Verification items for the finished model (mm, model axes). Face numbers are marked on the shaded views. A direction names the side the tool comes from. Give positions to 0.01 mm unless a question says otherwise; leave off trailing zeros. Write each loop counter-clockwise with the first axis right and the second up, starting at its lowest first coordinate (ties: lowest second). Pieces come first, ordered by that corner, then holes. Notation, with made-up numbers: (43.25, 46.5) -> (71.25, 46.5) arc R10 cw to (71.25, 60.5) -> close; hole circle Ø9 at (19, 47). An arc over 180 degrees is marked (long way). Answer as CSV lines item,"result".
```python
from build123d import *

# Parameters (mm, degrees)
BOSS_EXTRUDE1_DEPTH = 10
SKETCH4_R           = 4
CUT_EXTRUDE1_DEPTH  = 11


with BuildPart() as part:
    # Sketch3 → Boss-Extrude1 (new body)
    with BuildSketch(Plane.XY):
        with BuildLine():
            Line((-13.081475452, 10.960155108), (-10.960155108, 8.838834765))
            Line((-10.960155108, 8.838834765), (-10.960155108, -8.838834765))
            Line((-10.960155108, -8.838834765), (-13.081475452, -10.960155108))
            ThreePointArc((-13.081475452, -10.960155108), (-13.081475452, -13.081475452), (-10.960155108, -13.081475452))
            Line((-10.960155108, -13.081475452), (-8.838834765, -10.960155108))
            Line((-8.838834765, -10.960155108), (8.838834765, -10.960155108))
            Line((8.838834765, -10.960155108), (10.960155108, -13.081475452))
            ThreePointArc((10.960155108, -13.081475452), (13.081475452, -13.081475452), (13.081475452, -10.960155108))
            Line((13.081475452, -10.960155108), (10.960155108, -8.838834765))
            Line((10.960155108, -8.838834765), (10.960155108, 8.838834765))
            Line((10.960155108, 8.838834765), (13.081475452, 10.960155108))
            ThreePointArc((13.081475452, 10.960155108), (13.081475452, 13.081475452), (10.960155108, 13.081475452))
            Line((10.960155108, 13.081475452), (8.838834765, 10.960155108))
            Line((8.838834765, 10.960155108), (-8.838834765, 10.960155108))
            Line((-8.838834765, 10.960155108), (-10.960155108, 13.081475452))
            ThreePointArc((-10.960155108, 13.081475452), (-13.081475452, 13.081475452), (-13.081475452, 10.960155108))
        make_face()
    extrude(amount=-BOSS_EXTRUDE1_DEPTH)

    # Sketch4 → Cut-Extrude1 (cut, through all)
    with BuildSketch(Plane.XY):
        Circle(SKETCH4_R)
    extrude(amount=-CUT_EXTRUDE1_DEPTH, mode=Mode.SUBTRACT)


solid = part.part
```
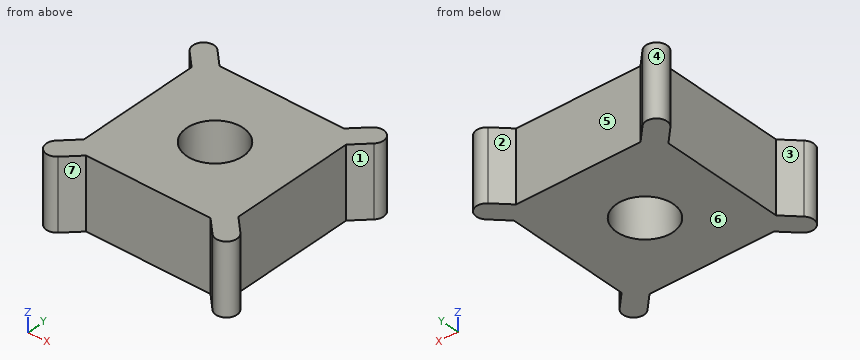
1) Section check A-A (y = 0). Record the boundary of the cut face in (x, z), and give its area (3 significant figures).
Reported:
outline,"(-10.96, -10) -> (-4, -10) -> (-4, 0) -> (-10.96, 0) -> close; (4, -10) -> (10.96, -10) -> (10.96, 0) -> (4, 0) -> close"
area,"139 mm²"
2) Tool access check on the marked faces 1, 2 and 3. Record the directions out of +Z, -Z, +X, -X, +Y, -Y that give a thin tool (end or side, any length) a straight path to the whole face; none if there is none.
Reported:
face 1,"+Z, -Z, +X"
face 2,"+Z, -Z, +Y"
face 3,"+Z, -Z, -X"
3) Section check B-B (z = -5). Record the boundary of the cut face in (x, y).
Reported:
outline,"(-13.08, -10.96) arc R1.5 ccw to (-10.96, -13.08) -> (-8.84, -10.96) -> (8.84, -10.96) -> (10.96, -13.08) arc R1.5 ccw to (13.08, -10.96) -> (10.96, -8.84) -> (10.96, 8.84) -> (13.08, 10.96) arc R1.5 ccw to (10.96, 13.08) -> (8.84, 10.96) -> (-8.84, 10.96) -> (-10.96, 13.08) arc R1.5 ccw to (-13.08, 10.96) -> (-10.96, 8.84) -> (-10.96, -8.84) -> close; hole circle Ø8 at (0, 0)"
4) Depth check by flat-ended pin: pin 1 (3 mm diameter, centred on y = 7.5, z = -1, fed in from -X); pin 2 (1.5 mm diameter, centred on y = -5.5, z = -8, fed in from -X); pin 3 (1 mm diameter, centred on y = -10.5, z = -5.5, fed in from -X). Enter the tip coordinate at first touch or a pass-through.
Reported:
pin 1,"x = -11.12"
pin 2,"x = -10.96"
pin 3,"x = -13.12"
5) Section check D-D (x = 5.5). Record the boundary of the cut face in (y, z).
Reported:
outline,"(-10.96, -10) -> (10.96, -10) -> (10.96, 0) -> (-10.96, 0) -> close"
6) Scan lines: line 1 along Y through (x, z) = (0, -2.25); line 2 along X through (y, z) = (-7, -6). Record each from-to range of solid material in increasing order.
Reported:
line 1,"-10.96 to -4, 4 to 10.96"
line 2,"-10.96 to 10.96"
7) Draft check along Y on the marked faces 4, 5, 6 and 7. Enter one of: +Y half, -Y half, draft (parallel to the pull), parting line (faces both ways), or undercut.
Reported:
face 4,"undercut"
face 5,"+Y half"
face 6,"draft"
face 7,"-Y half"
